Can you work these out from the model? Positions are in its coordinate system, mm. A direction names the side the tool comes from. Coordinates: 2 decimals unless noted, no trailing zeros. Write each loop counter-clockwise with the first axis right and the second up, starting at its lowest first coordinate (ties: lowest second). Pieces come first, ordered by that corner, then holes.
```python
from build123d import *

# Parameters (mm, degrees)
SKETCH1_R                                  = 3.302
SKETCH1_R_2                                = 0.8
SKETCH1_R_3                                = 1.8288
PLATE_DEPTH                                = 6.35
WEIGHT_SAVING_CUTS_DEPTH                   = 3.81
WEIGHT_SAVING_CUT_FILLETS_R                = 7.112
WEIGHT_SAVING_CUT_FILLETS_OF_WEIGHT_SAVI_R = 7.112


with BuildPart() as part:
    # Sketch1 → Plate (new body)
    with BuildSketch(Plane.XY):
        with BuildLine():
            ThreePointArc((-92.41454916, 90.390466105), (-90.529528169, 87.293813231), (-89.872400011, 83.728599949))
            Line((-89.872400011, 83.728599949), (-89.872400011, -113.728599949))
            Line((-89.872400011, -113.728599949), (-13.969765558, -113.728599949))
            ThreePointArc((-13.969765558, -113.728599949), (-9.672797049, -115.173448492), (-7.12174212, -118.920933572))
            Line((-7.12174212, -118.920933572), (-6.06808826, -122.679631657))
            ThreePointArc((-6.06808826, -122.679631657), (-3.807578113, -126.000308116), (0, -127.280599949))
            Line((0, -127.280599949), (0, -124.280599949))
            ThreePointArc((0, -124.280599949), (-3.302, -120.978599949), (0, -117.676599949))
            Line((0, -117.676599949), (0, 113.728599949))
            Line((0, 113.728599949), (-70.872400011, 113.728599949))
            ThreePointArc((-70.872400011, 113.728599949), (-75.894449931, 115.081113921), (-79.558021314, 118.772797028))
            Line((-79.558021314, 118.772797028), (-86.39815149, 130.760921117))
            ThreePointArc((-86.39815149, 130.760921117), (-88.915607296, 132.662483019), (-92.02827915, 132.147900342))
            Line((-92.02827915, 132.147900342), (-106.211434698, 123.072672373))
            ThreePointArc((-106.211434698, 123.072672373), (-110.686595056, 116.074115319), (-108.260147064, 108.129355334))
            Line((-108.260147064, 108.129355334), (-92.41454916, 90.390466105))
        make_face()
        with Locations((-100.872400011, 114.728599949)):
            Circle(SKETCH1_R, mode=Mode.SUBTRACT)
        with Locations((-82.452600011, 117.728599949)):
            Circle(SKETCH1_R_2, mode=Mode.SUBTRACT)
        with Locations((-83.72, -56.750000051)):
            Circle(SKETCH1_R_3, mode=Mode.SUBTRACT)
        with Locations((-83.72, 56.902399949)):
            Circle(SKETCH1_R_3, mode=Mode.SUBTRACT)
    plate = extrude(amount=-PLATE_DEPTH)

    # Plate Mirror: Plate across plane
    add(plate.mirror(Plane(origin=(0, 0, 0), x_dir=(0, 0, 1), z_dir=(1, 0, 0))))

    # Sketch2 → Weight Saving Cuts (cut)
    with BuildSketch(Plane.XY.offset(-6.35)):
        Polygon((-4, -52.750000051), (-71.028738776, -52.750000051), (-4, -7.31425078), align=None)
        Polygon((-4, -110.347555783), (-68.648884958, -60.750000051), (-4, -60.750000051), align=None)
        Polygon((-23.163651007, -105.728599949), (-79.72, -105.728599949), (-79.72, -62.33950402), align=None)
        Polygon((-79.91, -49.564541674), (-12.410965189, -3.81), (-79.91, -3.81), align=None)
        Polygon((-12.284928228, 3.81), (-79.91, 49.711527156), (-79.91, 3.81), align=None)
        Polygon((-4, 53.092399949), (-71.322809123, 53.092399949), (-4, 7.396038078), align=None)
        Polygon((-21.998091507, 64.902399949), (-75.72, 95.699068062), (-75.72, 64.902399949), align=None)
        Polygon((-4, 106.89580016), (-4, 63.806088559), (-79.165973641, 106.89580016), align=None)
    weight_saving_cuts = extrude(amount=WEIGHT_SAVING_CUTS_DEPTH, mode=Mode.SUBTRACT)

    # Weight Saving Cut Fillets
    weight_saving_cut_fillets_edges = [part.edges().sort_by_distance(p)[0] for p in [
        (-71.028738776, -52.750000051, -4.445),
        (-4, -52.750000051, -4.445),
        (-4, -7.31425078, -4.445),
        (-68.648884958, -60.750000051, -4.445),
        (-4, -110.347555783, -4.445),
        (-4, -60.750000051, -4.445),
        (-79.72, -105.728599949, -4.445),
        (-23.163651007, -105.728599949, -4.445),
        (-79.72, -62.33950402, -4.445),
        (-79.91, -49.564541674, -4.445),
        (-12.410965189, -3.81, -4.445),
        (-79.91, -3.81, -4.445),
        (-12.284928228, 3.81, -4.445),
        (-79.91, 49.711527156, -4.445),
        (-79.91, 3.81, -4.445),
        (-4, 53.092399949, -4.445),
        (-71.322809123, 53.092399949, -4.445),
        (-4, 7.396038078, -4.445),
        (-21.998091507, 64.902399949, -4.445),
        (-75.72, 95.699068062, -4.445),
        (-75.72, 64.902399949, -4.445),
        (-4, 63.806088559, -4.445),
        (-4, 106.89580016, -4.445),
        (-79.165973641, 106.89580016, -4.445),
    ]]
    fillet(weight_saving_cut_fillets_edges, radius=WEIGHT_SAVING_CUT_FILLETS_R)

    # Weight Saving Mirror: Weight Saving Cuts across plane
    add(weight_saving_cuts.mirror(Plane(origin=(0, 0, 0), x_dir=(0, 0, 1), z_dir=(1, 0, 0))), mode=Mode.SUBTRACT)

    # Weight Saving Cut Fillets of Weight Savi
    weight_saving_cut_fillets_of_weight_savi_edges = [part.edges().sort_by_distance(p)[0] for p in [
        (71.028738776, -52.750000051, -4.445),
        (4, -52.750000051, -4.445),
        (4, -7.31425078, -4.445),
        (68.648884958, -60.750000051, -4.445),
        (4, -110.347555783, -4.445),
        (4, -60.750000051, -4.445),
        (79.72, -105.728599949, -4.445),
        (23.163651007, -105.728599949, -4.445),
        (79.72, -62.33950402, -4.445),
        (79.91, -49.564541674, -4.445),
        (12.410965189, -3.81, -4.445),
        (79.91, -3.81, -4.445),
        (12.284928228, 3.81, -4.445),
        (79.91, 49.711527156, -4.445),
        (79.91, 3.81, -4.445),
        (4, 53.092399949, -4.445),
        (71.322809123, 53.092399949, -4.445),
        (4, 7.396038078, -4.445),
        (21.998091507, 64.902399949, -4.445),
        (75.72, 95.699068062, -4.445),
        (75.72, 64.902399949, -4.445),
        (4, 63.806088559, -4.445),
        (4, 106.89580016, -4.445),
        (79.165973641, 106.89580016, -4.445),
    ]]
    fillet(weight_saving_cut_fillets_of_weight_savi_edges, radius=WEIGHT_SAVING_CUT_FILLETS_OF_WEIGHT_SAVI_R)


solid = part.part
```
1. If we section it at A-A, the plane z = -1: Count the separate pieces of the cut face and the enclosed holes in it, plus the area to 3 significant figures.
2. We'd pull the mould along Y, two halves only. Please class faces 1 (the face through (-90.548, 87.341, -3.131)), 2 (the face through (-73.58, 66.93, -4.42)), 3 (the face through (-99.021, 127.674, -3.131)), 4 (the face through (-7.46, 69.98, -4.42)): released by +Y, released by -Y, zero draft, split by the parting line, or undercut.
3. Which directions (+Z, -Z, +X, -X, +Y, -Y) give clear straight access to the entire face, cutting with the end or side of a thin tool? Please do faces 5 (the face through (88.87, 132.65, -3.13)), 6 (the face through (24, 38, -2.54)).
4. If we section it at B-B, the plane y = 25: List the corners of the cut face in (x, z) for me.
5. If we section it at C-C, the plane y = -85: List the corners of the cut face in (x, z) for me, plus the area to 3 significant figures.
6. I'm going to push flat-ended pins straight in: P1, Ø6, axis at x = -26.5, y = -95, coming from the +Z side; P2, Ø1.9, axis at y = 29.5, z = -5, coming from the -X side; P3, Ø3, axis at x = -21, y = 40, coming from the -Z side; P4, Ø1.5, axis at x = 2, z = -2.5, coming from the -Y side. Where does each tip first touch, or does it pass through?
7. If I drill on L1, parallel to X at y = -56.75, z = -5; L2, parallel to Y at x = 83.72, z = -3.75; L3, parallel to Y at x = 69.5, z = -3.75, over which ranges is the centre line in solid material (lowest first)?
Answers:
1. separate pieces: 1
1. enclosed holes: 9
1. area: 42,400 mm2
2. face 1: released by -Y
2. face 2: undercut
2. face 3: released by +Y
2. face 4: undercut
3. face 5: +Z, -Z, +Y
3. face 6: -Z
4. outline: (-89.87, -6.35) - (-79.91, -6.35) - (-79.91, -2.54) - (-43.5, -2.54) - (-43.5, -6.35) - (-29.94, -6.35) - (-29.94, -2.54) - (-4, -2.54) - (-4, -6.35) - (4, -6.35) - (4, -2.54) - (29.94, -2.54) - (29.94, -6.35) - (43.5, -6.35) - (43.5, -2.54) - (79.91, -2.54) - (79.91, -6.35) - (89.87, -6.35) - (89.87, 0) - (-89.87, 0) - close
5. outline: (-89.87, -6.35) - (-79.72, -6.35) - (-79.72, -2.54) - (-50.18, -2.54) - (-50.18, -6.35) - (-37.04, -6.35) - (-37.04, -2.54) - (-4, -2.54) - (-4, -6.35) - (4, -6.35) - (4, -2.54) - (37.04, -2.54) - (37.04, -6.35) - (50.18, -6.35) - (50.18, -2.54) - (79.72, -2.54) - (79.72, -6.35) - (89.87, -6.35) - (89.87, 0) - (-89.87, 0) - close
5. area: 665 mm2
6. P1: stops at z = 0
6. P2: stops at x = -89.87
6. P3: stops at z = -2.54
6. P4: stops at y = -127.16
7. L1: x = -89.87 to -85.55, -81.89 to 81.89, 85.55 to 89.87
7. L2: y = -113.73 to -58.58, -54.92 to 55.07, 58.73 to 126.07
7. L3: y = -113.73 to -105.73, -70.36 to -42.45, -3.81 to 3.81, 42.59 to 64.96, 90.48 to 113.73
